The listing builds one solid part. Answer for the finished solid, in the listing's coordinates (mm). Face numbers are marked on the shaded views. A direction names the side the tool comes from. Round coordinates to 2 decimals unless told otherwise and drop trailing zeros. Write each loop counter-clockwise with the first axis right and the second up, starting at its lowest first coordinate (ties: lowest second). Pieces come first, ordered by that corner, then holes. Notation, with made-up numbers: (48.25, 49.5) - (103.25, 49.5) arc R20 cw to (103.25, 77.5) - close; hole circle Ø9 at (19.5, 21). An arc over 180 degrees is marked (long way). Return JSON: item names as keys, results as strings. Group by question number.
(1) Determine the mould class of the marked faces 1, 2, 3 and 4 for opening direction Y: +Y half, -Y half, draft (parallel to the pull), parting line (faces both ways), or undercut.
(2) Find the intervals of material crossed by line 1 along Y through (x, z) = (5, 0.5); line 2 along Y through (x, z) = (-1.5, 2.5); line 3 along Z through (x, y) = (2.25, 16), in increasing order. Write a range as [from, to].
(3) Section D-D, the plane y = 5.25 is taken. Write down the section's boundary in (x, z).
(4) Section A-A, the plane y = 11.25 is taken. Write down the section's boundary in (x, z).
(5) Section C-C, the plane x = 1 is taken. Write down the section's boundary in (y, z).
(6) Which of the six approach directions +Z, -Z, +X, -X, +Y, -Y give full straight-line access (tool end or side, diameter ignored) to the marked faces 5, 6 and 7?
(7) Each of these flat-tipped pins is pushed along its axis until it touches: pin 1 (5 mm diameter, centred on x = -1.5, y = 2.5, fed in from +Z); pin 2 (1.5 mm diameter, centred on x = 2.5, y = 12.5, fed in from +Z); pin 3 (2 mm diameter, centred on x = 4.5, z = 4, fed in from +Y). Where does it stop, or does it pass through?
(8) Section B-B, the plane z = 0 is taken. Write down the section's boundary in (x, y) (3 decimals).
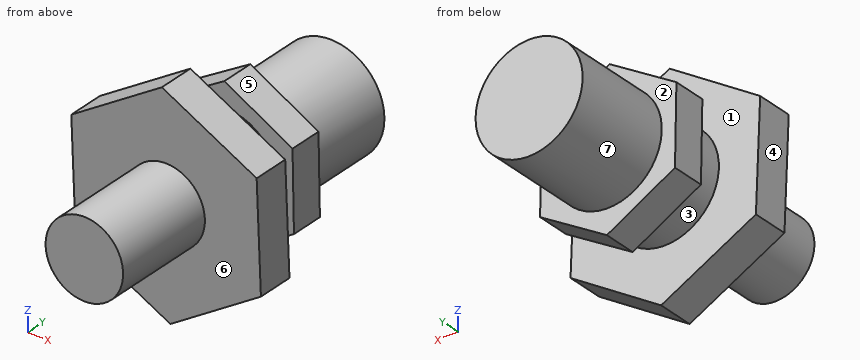
Autodesk Inventor part; units mm, degrees
ref_plane "YZ Plane" through (0, 0, 0) normal (1, 0, 0) x (0, 1, 0)
ref_plane "XZ Plane" through (0, 0, 0) normal (0, 1, 0) x (-1, 0, 0)
ref_plane "XY Plane" through (0, 0, 0) normal (0, 0, 1) x (1, 0, 0)
sketch "Sketch1" plane through (0, 0, 0) normal (0, 1, 0) x (-1, 0, 0)
  circle A0 centre (0, 0) radius 2.3
  dimension "d0" = 4.6
extrude "Extrusion1" add sketch "Sketch1" along normal blind 6.3
sketch "Sketch2" plane through (0, 6.3, 0) normal (0, 1, 0) x (1, 0, 0)
  circle A0 centre (0, 0) radius 2.3
  line L0 (5.6221, 2.954) -> (5.3692, -3.3919)
  line L1 (5.3692, -3.3919) -> (-0.2528, -6.3458)
  line L2 (-0.2528, -6.3458) -> (-5.6221, -2.954)
  line L3 (-5.6221, -2.954) -> (-5.3692, 3.3919)
  line L4 (-5.3692, 3.3919) -> (0.2528, 6.3458)
  line L5 (0.2528, 6.3458) -> (5.6221, 2.954)
  dimension "d10" = 11
extrude "Extrusion2" add sketch "Sketch2" along normal blind 2.2 contours A0 | L0 L1 L2 L3 L4 L5
sketch "Sketch3" plane through (0, 8.5, 0) normal (0, 1, 0) x (1, 0, 0)
  circle A0 centre (0, 0) radius 3.175
  dimension "d6" = 6.35
extrude "Extrusion3" add sketch "Sketch3" along normal blind 2.4
sketch "Sketch4" plane through (0, 10.9, 0) normal (0, 1, 0) x (1, 0, 0)
  circle A0 centre (0, 0) radius 3.175
  line L0 (4.0415, 2.236) -> (3.9572, -2.3821)
  line L1 (3.9572, -2.3821) -> (-0.0844, -4.618)
  line L2 (-0.0844, -4.618) -> (-4.0415, -2.236)
  line L3 (-4.0415, -2.236) -> (-3.9572, 2.3821)
  line L4 (-3.9572, 2.3821) -> (0.0844, 4.618)
  line L5 (0.0844, 4.618) -> (4.0415, 2.236)
  dimension "d9" = 8
extrude "Extrusion4" add sketch "Sketch4" along normal blind 2 contours A0 | L0 L1 L2 L3 L4 L5
sketch "Sketch5" plane through (0, 12.9, 0) normal (0, 1, 0) x (1, 0, 0)
  circle A0 centre (0, 0) radius 3.175
  dimension "d13" = 6.35
extrude "Extrusion5" add sketch "Sketch5" along normal blind 6.1
properties part number "SMA_Bulkhead"
Working result:
{
 "1": {"face 1": "undercut", "face 2": "+Y half", "face 3": "undercut", "face 4": "draft"},
 "2": {"line 1": "y = [6.3, 8.5]", "line 2": "y = [6.3, 19]", "line 3": "z = [-2.24, 2.24]"},
 "3": {"outline": "circle Ø4.6 at (0, 0)"},
 "4": {"outline": "(-4.04, 2.24) - (-3.96, -2.38) - (0.08, -4.62) - (4.04, -2.24) - (3.96, 2.38) - (-0.08, 4.62) - close"},
 "5": {"outline": "(0, -2.07) - (6.3, -2.07) - (6.3, -5.87) - (8.5, -5.87) - (8.5, -3.01) - (10.9, -3.01) - (10.9, -4.07) - (12.9, -4.07) - (12.9, -3.01) - (19, -3.01) - (19, 3.01) - (12.9, 3.01) - (12.9, 4.02) - (10.9, 4.02) - (10.9, 3.01) - (8.5, 3.01) - (8.5, 5.69) - (6.3, 5.69) - (6.3, 2.07) - (0, 2.07) - close"},
 "6": {"face 5": "+Z, +X, +Y", "face 6": "-Y", "face 7": "+Y"},
 "7": {"pin 1": "stops at z = 2.3", "pin 2": "stops at z = 3.6", "pin 3": "stops at y = 8.5"},
 "8": {"outline": "(-5.504, 6.3) - (-2.3, 6.3) - (-2.3, 0) - (2.3, 0) - (2.3, 6.3) - (5.504, 6.3) - (5.504, 8.5) - (3.175, 8.5) - (3.175, 10.9) - (4.001, 10.9) - (4.001, 12.9) - (3.175, 12.9) - (3.175, 19) - (-3.175, 19) - (-3.175, 12.9) - (-4.001, 12.9) - (-4.001, 10.9) - (-3.175, 10.9) - (-3.175, 8.5) - (-5.504, 8.5) - close"}
}
